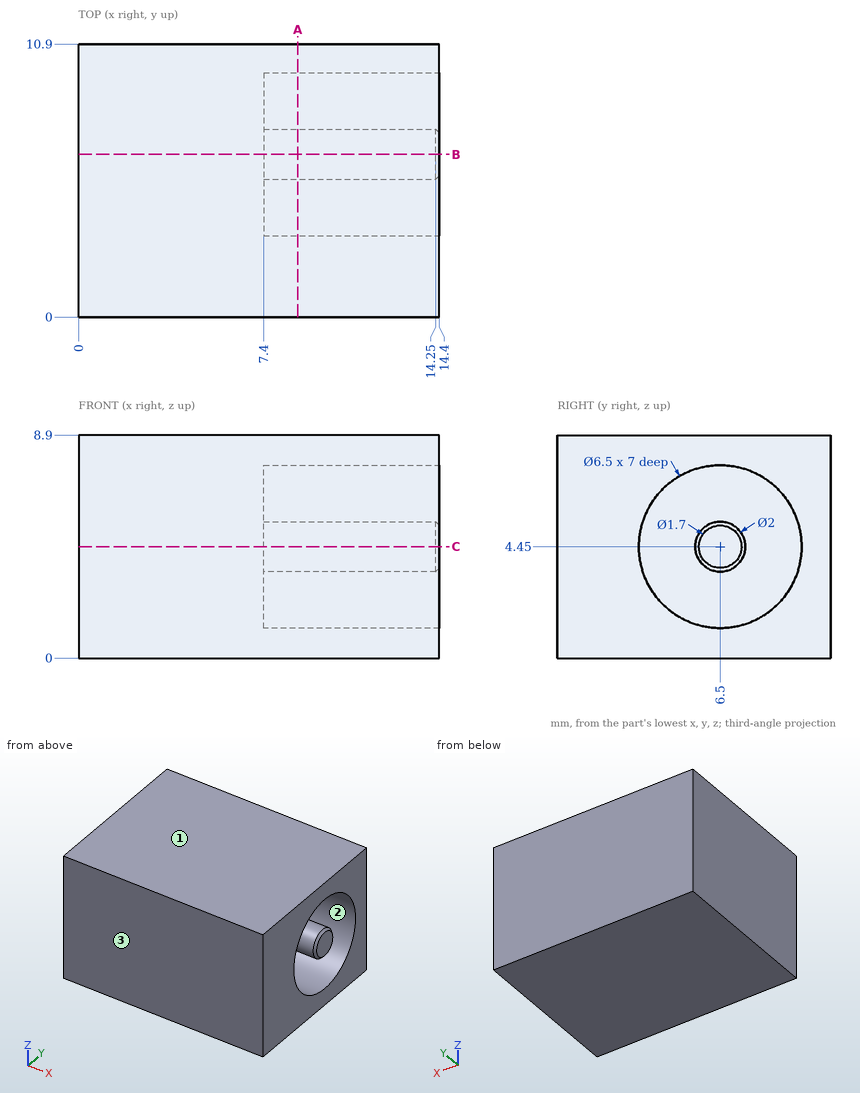
Design review of the part shown in the three views and the two pictorial views. Dimensions are in mm from the part's minimum x, y and z. Give positions to 0.01 mm unless a question says otherwise; leave off trailing zeros. Write each loop counter-clockwise with the first axis right and the second up, starting at its lowest first coordinate (ties: lowest second). Pieces come first, ordered by that corner, then holes. Notation, with made-up numbers: M -13.5,-7.5 L 21.5,-7.5 A22 cw 21.5,3.5 Z; hole C 18.5,79.25 d2. An arc over 180 degrees is marked long. Answer in a Markdown table with one row per item.
Item 1: Draft analysis for pull direction Y (two halves, no side actions). For the marked faces 1, 2 and 3, state which applies: +Y half, -Y half, draft (parallel to the pull), parting line (faces both ways), or undercut.
Check sheet entries:
| item | result |
|---|---|
| face 1 | draft |
| face 2 | undercut |
| face 3 | -Y half |
Item 2: For line 1 along Y through (x, z) = (11, 4.45); line 2 along Z through (x, y) = (11.25, 6.5); line 3 along X through (y, z) = (5.5, 5.75), list the stretches that pass through material, from the lowest coordinate up.
Check sheet entries:
| item | result |
|---|---|
| line 1 | 0 to 3.25, 5.5 to 7.5, 9.75 to 10.9 |
| line 2 | 0 to 1.2, 3.45 to 5.45, 7.7 to 8.9 |
| line 3 | 0 to 7.4 |
Item 3: Add section A-A on x = 8.75. Give the boundary of the cut face in (y, z), plus the area to 3 significant figures.
Check sheet entries:
| item | result |
|---|---|
| outline | M 0,0 L 10.9,0 L 10.9,8.9 L 0,8.9 Z; C 6.5,4.45 d2; hole C 6.5,4.45 d6.5 |
| area | 67.0 mm2 |
Item 4: For P1, Ø1, axis at x = 5, y = 5, coming from the -Z side, flat-tipped, find the tip position at first contact; note if it passes through.
Check sheet entries:
| item | result |
|---|---|
| P1 | z = 0 |
Item 5: Add section C-C on z = 4.45. Give the boundary of the cut face in (x, y), plus the area to 3 significant figures.
Check sheet entries:
| item | result |
|---|---|
| outline | M 0,0 L 14.4,0 L 14.4,3.25 L 7.4,3.25 L 7.4,5.5 L 14.25,5.5 L 14.4,5.65 L 14.4,7.35 L 14.25,7.5 L 7.4,7.5 L 7.4,9.75 L 14.4,9.75 L 14.4,10.9 L 0,10.9 Z |
| area | 125 mm2 |
Item 6: Add section B-B on y = 6.5. Give the boundary of the cut face in (x, z).
Check sheet entries:
| item | result |
|---|---|
| outline | M 0,0 L 14.4,0 L 14.4,1.2 L 7.4,1.2 L 7.4,3.45 L 14.25,3.45 L 14.4,3.6 L 14.4,5.3 L 14.25,5.45 L 7.4,5.45 L 7.4,7.7 L 14.4,7.7 L 14.4,8.9 L 0,8.9 Z |
